```python
from build123d import *

# Parameters (mm, degrees)
SKETCH_1_R      = 1.25
SKETCH_1_R_2    = 1.5
SKETCH_1_W      = 12.000960833
SKETCH_1_H      = 22.8
EXTRUDE_1_DEPTH = 3


with BuildPart() as part:
    # 草圖1 → 填料-伸長1 (new body)
    with BuildSketch(Plane.XY):
        with BuildLine():
            Line((224.799401664, 107.985882496), (221.799401664, 107.985882496))
            Line((221.799401664, 107.985882496), (221.799401664, 119.985882496))
            Line((221.799401664, 119.985882496), (224.799369028, 119.985882496))
            Line((224.799369028, 119.985882496), (224.799401664, 127.645063489))
            ThreePointArc((224.799401664, 127.645063489), (223.796832359, 129.736024952), (221.603142855, 130.487684059))
            Line((221.603142855, 130.487684059), (203.993498606, 130.487684059))
            ThreePointArc((203.993498606, 130.487684059), (201.928341095, 129.663767205), (200.997480004, 127.64455643))
            Line((200.997480004, 127.64455643), (200.997480004, 119.985882496))
            Line((200.997480004, 119.985882496), (203.997720212, 119.985882496))
            Line((203.997720212, 119.985882496), (203.997720212, 107.985882496))
            Line((203.997720212, 107.985882496), (200.997480004, 107.985882496))
            Line((200.997480004, 107.985882496), (200.997480004, 90.984521316))
            ThreePointArc((200.997480004, 90.984521316), (201.841197388, 88.898693406), (203.897756422, 87.985949173))
            Line((203.897756422, 87.985949173), (221.799361625, 87.987966928))
            ThreePointArc((221.799361625, 87.987966928), (223.920611625, 88.866716927), (224.799361625, 90.987966928))
            Line((224.799361625, 90.987966928), (224.799401664, 107.985882496))
        make_face()
        with Locations((204.297950444, 127.688016928)):
            Circle(SKETCH_1_R, mode=Mode.SUBTRACT)
        with Locations((221.299311625, 127.688016928)):
            Circle(SKETCH_1_R, mode=Mode.SUBTRACT)
        with Locations((221.299311625, 100.485839038)):
            Circle(SKETCH_1_R, mode=Mode.SUBTRACT)
        with Locations((221.849455668, 90.985078375)):
            Circle(SKETCH_1_R_2, mode=Mode.SUBTRACT)
        with Locations((203.748006411, 90.985078375)):
            Circle(SKETCH_1_R_2, mode=Mode.SUBTRACT)
        with Locations((204.297950444, 100.485839038)):
            Circle(SKETCH_1_R, mode=Mode.SUBTRACT)
        with Locations((212.79832073, 113.885949173)):
            Rectangle(SKETCH_1_W, SKETCH_1_H, mode=Mode.SUBTRACT)
    extrude(amount=EXTRUDE_1_DEPTH)


solid = part.part
```
Input: part model. Units: mm. Frame: model coordinates. A direction names the side the tool comes from. Give positions to 0.01 mm unless a question says otherwise; leave off trailing zeros. Loops run counter-clockwise (first coordinate to the right, second up) from the corner with the lowest first, then second, coordinate; pieces in that order, holes last. Notation, with made-up numbers: M -11.5,78.25 L 18.5,78.25 A20 ccw 18.5,116.25 Z; hole C 53.5,51 d7. An arc over 180 degrees is marked long. Answer as CSV lines item,"result". Start each with the question number.
1. Pull-direction query (X, two-part tool) for faces 1 (the face through (213, 125.286, 1)), 2 (the face through (223, 107.986, 1)), 3 (the face through (222.454, 100.007, 1.479)), 4 (the face through (200.997, 124, 1)); classes: released by +X, released by -X, zero draft, split by the parting line, or undercut.
2. Reachability of faces 5 (the face through (203, 107.986, 1)), 6 (the face through (223, 119.986, 1)), 7 (the face through (206.798, 114, 1)), 8 (the face through (201.952, 129.686, 1.479)) from +Z, -Z, +X, -X, +Y, -Y: full face, straight path, thin tool, end or side. Return the list, or none.
3. Pin query (flat end, axial travel): P1, Ø1.5, axis at x = 211.5, z = 1.5, coming from the +Y side; P2, Ø0.9, axis at y = 113.5, z = 1, coming from the +X side; P3, Ø1.5, axis at y = 112.5, z = 2, coming from the -X side. Return the tip coordinate at first contact, or that it passes through.
4. Section D-D on y = 124. Return loops of the section in (x, z).
5. Line query: L1, parallel to Y at x = 212, z = 2; L2, parallel to X at y = 124, z = 0.2; L3, parallel to X at y = 119, z = 0.9. Output: solid intervals per line, ascending.
6. Section B-B on y = 128.5. Return loops of the section in (x, z).
7. Section A-A on x = 215.75. Return loops of the section in (y, z), plus the area to 3 significant figures.
8. Section C-C on z = 1. Return loops of the section in (x, y).
Computed values:
1,face 1,"undercut"
1,face 2,"zero draft"
1,face 3,"undercut"
1,face 4,"released by -X"
2,face 5,"+Z, -Z, -X"
2,face 6,"+Z, -Z, +X"
2,face 7,"+Z, -Z"
2,face 8,"+Z, -Z, -X, +Y"
3,P1,"stops at y = 130.49"
3,P2,"stops at x = 221.8"
3,P3,"stops at x = 204"
4,outline,"M 201,0 L 206.8,0 L 206.8,3 L 201,3 Z; M 218.8,0 L 224.8,0 L 224.8,3 L 218.8,3 Z"
5,L1,"y = 87.99 to 102.49, 125.29 to 130.49"
5,L2,"x = 201 to 206.8, 218.8 to 224.8"
5,L3,"x = 204 to 206.8, 218.8 to 221.8"
6,outline,"M 201.17,0 L 203.35,0 L 203.35,3 L 201.17,3 Z; M 205.25,0 L 220.35,0 L 220.35,3 L 205.25,3 Z; M 222.25,0 L 224.63,0 L 224.63,3 L 222.25,3 Z"
7,outline,"M 87.99,0 L 102.49,0 L 102.49,3 L 87.99,3 Z; M 125.29,0 L 130.49,0 L 130.49,3 L 125.29,3 Z"
7,area,"59.1 mm²"
8,outline,"M 201,90.98 A3 ccw 203.9,87.99 L 221.8,87.99 A3 ccw 224.8,90.99 L 224.8,107.99 L 221.8,107.99 L 221.8,119.99 L 224.8,119.99 L 224.8,127.65 A3 ccw 221.6,130.49 L 203.99,130.49 A3 ccw 201,127.64 L 201,119.99 L 204,119.99 L 204,107.99 L 201,107.99 Z; hole C 203.75,90.99 d3; hole C 204.3,100.49 d2.5; hole C 204.3,127.69 d2.5; hole M 206.8,102.49 L 218.8,102.49 L 218.8,125.29 L 206.8,125.29 Z; hole C 221.3,100.49 d2.5; hole C 221.3,127.69 d2.5; hole C 221.85,90.99 d3"
